Could you check a few things on this model? Use its own coordinates, in mm. Face numbers are marked on the shaded views. A direction names the side the tool comes from. Give positions to 0.01 mm unless a question says otherwise; leave off trailing zeros. Loops run counter-clockwise (first coordinate to the right, second up) from the corner with the lowest first, then second, coordinate; pieces in that order, holes last. Notation, with made-up numbers: (68.25, 73.5) - (117.25, 73.5) arc R13 cw to (117.25, 80.5) - close; hole circle Ø5 at (59.5, 23). An arc over 180 degrees is marked (long way). One line per item, written item: value. Start each with the question number.
Q1. If we mould it in two halves opening along Z, with no side actions, what happens to the marked faces 1, 2, 3 and 4? For each: released by +Z, released by -Z, zero draft, split by the parting line, or undercut.
Q2. I want a section at B-B (z = 12.5). Please give me the cut outline in (x, y).
Q3. For the marked faces 5, 6, 7, 8 and 9, which set-ups out of +Z, -Z, +X, -X, +Y, -Y let a thin tool reach every point of the face, with its end or its side?
Q4. I want a section at D-D (x = -44). Please give me the cut outline in (y, z), then the cut area to 3 significant figures.
Q5. I want a section at C-C (y = -27). Please give me the cut outline in (x, z).
Q6. I'm going to push flat-ended pins straight in: P1, Ø5, axis at y = 14, z = 10.5, coming from the -X side; P2, Ø5, axis at x = -13, y = -0.5, coming from the -Z side; P3, Ø3, axis at x = -36, z = -16, coming from the +Y side. Where does each tip first touch, or does it pass through?
Q7. I want a section at A-A (x = -12.5). Please give me the cut outline in (y, z).
Q8. If I drill on line 1 (Y direction, x = -17, z = 24.5); line 2 (Z direction, x = -44, y = -2); line 3 (Y direction, x = -43, z = 34), over which ranges is the centre line in solid material (lowest first)? Write a range as from..to.
```python
from build123d import *

# Parameters (mm, degrees)
F0_W     = 50
F0_H     = 50
F1_DEPTH = 50
F2_R     = 5.653003
F3_DEPTH = 25
F4_R     = 10.570293
F5_DEPTH = 10
F6_W     = 10
F6_H     = 10
F7_DEPTH = 25


with BuildPart() as f1:
    # F0 (on Front) → F1 (new body)
    with BuildSketch(Plane.XZ):
        with Locations((-25, 25)):
            Rectangle(F0_W, F0_H)
    extrude(amount=F1_DEPTH)

    # F2 (on face) → F3 (join)
    with BuildSketch(Plane(origin=(0, 0, 0), x_dir=(1, 0, 0), z_dir=(0, 0, -1))):
        with Locations((-32.565601, 25.707576)):
            Circle(F2_R)
    extrude(amount=F3_DEPTH)

    # F4 (on face) → F5 (cut)
    with BuildSketch(Plane(origin=(-50, 0, 0), x_dir=(0, -1, 0), z_dir=(-1, 0, 0))):
        with Locations((25.992477, 27.822873)):
            Circle(F4_R)
    extrude(amount=-F5_DEPTH, mode=Mode.SUBTRACT)

    # F6 (on face) → F7 (join)
    with BuildSketch(Plane(origin=(0, 0, 0), x_dir=(-1, 0, 0), z_dir=(0, 1, 0))):
        with Locations((10.811531, 10.130358)):
            Rectangle(F6_W, F6_H)
    extrude(amount=F7_DEPTH)


solid = f1.part
```
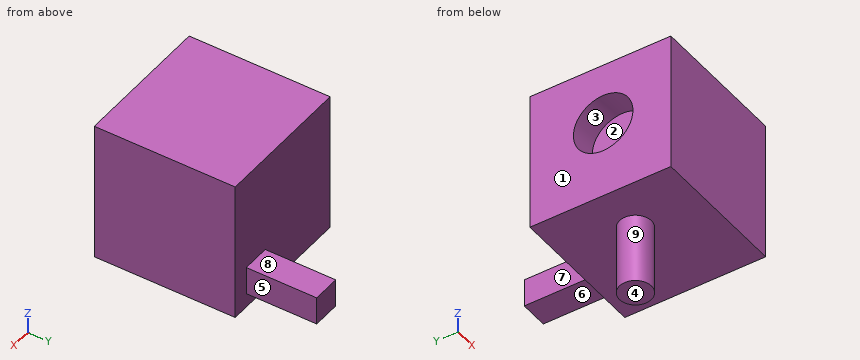
Worked answers:
1. face 1: zero draft
1. face 2: undercut
1. face 3: undercut
1. face 4: released by -Z
2. outline: (-50, -50) - (0, -50) - (0, 0) - (-5.81, 0) - (-5.81, 25) - (-15.81, 25) - (-15.81, 0) - (-50, 0) - close
3. face 5: +Z, -Z, +X, +Y
3. face 6: -Z, +X, -X, +Y
3. face 7: +Z, -Z, -X, +Y
3. face 8: +Z, +X, -X, +Y
3. face 9: -Z
4. outline: (-50, 0) - (0, 0) - (0, 50) - (-50, 50) - close; hole circle Ø21.14 at (-25.99, 27.82)
4. area: 2,150 mm²
5. outline: (-50, 0) - (-38.07, 0) - (-38.07, -25) - (-27.06, -25) - (-27.06, 0) - (0, 0) - (0, 50) - (-50, 50) - (-50, 38.35) - (-40, 38.35) - (-40, 17.3) - (-50, 17.3) - close
6. P1: stops at x = -15.81
6. P2: stops at z = 0
6. P3: stops at y = -20.4
7. outline: (-50, 0) - (0, 0) - (0, 5.13) - (25, 5.13) - (25, 15.13) - (0, 15.13) - (0, 50) - (-50, 50) - close
8. line 1: y = -50..0
8. line 2: z = 0..50
8. line 3: y = -50..-34.57, -17.41..0
